from build123d import *

# Parameters (mm, degrees)
F0_W     = 6.5
F0_H     = 17
F1_DEPTH = 1
F0_R     = 12.5
F2_DEPTH = 2


with BuildPart() as f1:
    # F0 (on Top) → F1 (new body)
    with BuildSketch(Plane.XY):
        with Locations((11.249999, -11.019001)):
            Rectangle(F0_W, F0_H)
    extrude(amount=F1_DEPTH)

    # F0 (on Top) → F2 (join)
    with BuildSketch(Plane.XY):
        with Locations((11.246626, -11.0498)):
            Circle(F0_R)
        with Locations((11.249999, -11.019001)):
            Rectangle(F0_W, F0_H, mode=Mode.SUBTRACT)
    extrude(amount=F2_DEPTH)


solid = f1.part
Build history of the part. All positions in model axes, mm. A direction names the side the tool comes from. Coordinates: 2 decimals unless noted, no trailing zeros. Order: outer loops, then holes, each group sorted by start corner. A loop starts at its lowest first (then second) coordinate and runs counter-clockwise, first axis right, second up. Notation, with made-up numbers: (-7.75, 52) - (-2.75, 52) arc R14 ccw to (-2.75, 79) - close; hole circle Ø5 at (-40, 26). An arc over 180 degrees is marked (long way). Put each result on its own line as item: value.
1. Saw through at B-B (x = 13). Write the cut outline in (y, z).
Answer sheet:
outline: (-23.43, 0) - (1.33, 0) - (1.33, 2) - (-2.52, 2) - (-2.52, 1) - (-19.52, 1) - (-19.52, 2) - (-23.43, 2) - close
2. Saw through at A-A (z = 1.65). Write the cut outline in (x, y), and give its area (3 significant figures).
Answer sheet:
outline: circle Ø25 at (11.25, -11.05); hole (8, -19.52) - (14.5, -19.52) - (14.5, -2.52) - (8, -2.52) - close
area: 380 mm^2
3. Tool access for faces 4 (the face through (11, -11, 0)), 5 (the face through (8, -11.1, 1.5)): list every direction of +Z, -Z, +X, -X, +Y, -Y with a clear straight run to the whole face (end or side of a thin tool).
Answer sheet:
face 4: -Z, +X, -X, +Y, -Y
face 5: +Z
4. Saw through at D-D (x = 18). Write the cut outline in (y, z), and give its area (3 significant figures).
Answer sheet:
outline: (-21.57, 0) - (-0.53, 0) - (-0.53, 2) - (-21.57, 2) - close
area: 42.1 mm^2
5. Pull direction Y, two halves, no side cores. Call faces 1 (the face through (11.2, -19.519, 1.5)), 2 (the face through (17, -11, 2)), 3 (the face through (-1.24, -10.5, 0.99)): pulls with the +Y half, pulls with the -Y half, needs draft (parallel to the pull), parting line crosses it, or undercut.
Answer sheet:
face 1: undercut
face 2: needs draft
face 3: parting line crosses it
6. Saw through at C-C (y = -12.75). Write the cut outline in (x, z), and give its area (3 significant figures).
Answer sheet:
outline: (-1.14, 0) - (23.63, 0) - (23.63, 2) - (14.5, 2) - (14.5, 1) - (8, 1) - (8, 2) - (-1.14, 2) - close
area: 43.0 mm^2
7. Drop flat-ended pins along their axis: P1, Ø1.1, axis at x = 11, z = 1.5, coming from the +Y side; P2, Ø1, axis at y = -18, z = 1.5, coming from the +X side; P3, Ø0.5, axis at y = -13, z = 1.5, coming from the -X side; P4, Ø3, axis at x = 10, y = -11.5, coming from the +Z side. Give the stop position or say it passes through.
Answer sheet:
P1: stops at y = 1.45
P2: stops at x = 21.95
P3: stops at x = -1.14
P4: stops at z = 1
8. Probe line 1 along Y through (x, z) = (11.5, 0.5); line 2 along X through (y, z) = (-13, 1.2); line 3 along X through (y, z) = (-6, 1.5). List the from-to ranges inside material, lowest first. Write a range as [from, to].
Answer sheet:
line 1: y = [-23.55, 1.45]
line 2: x = [-1.1, 8], [14.5, 23.59]
line 3: x = [-0.19, 8], [14.5, 22.68]
